Design review of the part built by this model. Coordinates are the model's own, in mm. Face numbers are marked on the shaded views. Give positions to 0.01 mm unless a question says otherwise; leave off trailing zeros. Write each loop counter-clockwise with the first axis right and the second up, starting at its lowest first coordinate (ties: lowest second). Pieces come first, ordered by that corner, then holes. Notation, with made-up numbers: (-10, -36.75) -> (13, -36.75) arc R25 ccw to (13, -22.75) -> close; hole circle Ø1 at (68.25, 70). An arc over 180 degrees is marked (long way). Return JSON: item names as keys, results as strings. Group by question number.
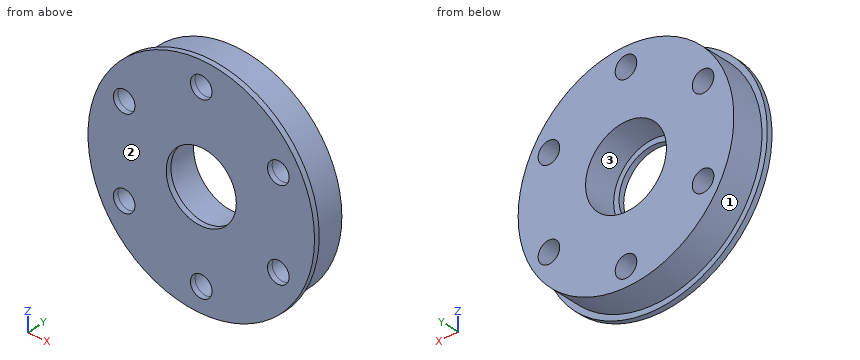
from build123d import *

# Parameters (mm, degrees)
SKETCH1_R           = 20
SKETCH1_R_2         = 7.5
BOSS_EXTRUDE1_DEPTH = 6
SKETCH2_R           = 2
CUT_EXTRUDE1_DEPTH  = 7
CIRPATTERN2_COUNT   = 6
SKETCH3_R           = 21
SKETCH3_R_2         = 6.5
SKETCH3_R_3         = 2
BOSS_EXTRUDE2_DEPTH = 1


with BuildPart() as part:
    # Sketch1 → Boss-Extrude1 (new body)
    with BuildSketch(Plane(origin=(0, 0, 0), x_dir=(1, 0, 0), z_dir=(0, 1, 0))):
        Circle(SKETCH1_R)
        Circle(SKETCH1_R_2, mode=Mode.SUBTRACT)
    extrude(amount=BOSS_EXTRUDE1_DEPTH)

    # Sketch2 → Cut-Extrude1 (cut, through all)
    with BuildSketch(Plane(origin=(0, 6, 0), x_dir=(1, 0, 0), z_dir=(0, 1, 0))):
        with Locations((0, 16.5)):
            Circle(SKETCH2_R)
    cut_extrude1 = extrude(amount=-CUT_EXTRUDE1_DEPTH, mode=Mode.SUBTRACT)

    # CirPattern2: Cut-Extrude1 ×6 about axis
    cirpattern2_axis = Axis((0, 0, 0), (0, 1, 0))
    for i in range(1, CIRPATTERN2_COUNT):
        add(cut_extrude1.rotate(cirpattern2_axis, i * 360 / CIRPATTERN2_COUNT), mode=Mode.SUBTRACT)

    # Sketch3 → Boss-Extrude2 (add)
    with BuildSketch(Plane(origin=(0, 0, 0), x_dir=(1, 0, 0), z_dir=(0, 1, 0))):
        Circle(SKETCH3_R)
        Circle(SKETCH3_R_2, mode=Mode.SUBTRACT)
        with Locations((-14.289419162, -8.25)):
            Circle(SKETCH3_R_3, mode=Mode.SUBTRACT)
        with Locations((0, -16.5)):
            Circle(SKETCH3_R_3, mode=Mode.SUBTRACT)
        with Locations((14.289419162, -8.25)):
            Circle(SKETCH3_R_3, mode=Mode.SUBTRACT)
        with Locations((14.289419162, 8.25)):
            Circle(SKETCH3_R_3, mode=Mode.SUBTRACT)
        with Locations((0, 16.5)):
            Circle(SKETCH3_R_3, mode=Mode.SUBTRACT)
        with Locations((-14.289419162, 8.25)):
            Circle(SKETCH3_R_3, mode=Mode.SUBTRACT)
    extrude(amount=-BOSS_EXTRUDE2_DEPTH)


solid = part.part
Q1. Mouldability with a two-part tool opening along Z and no side actions: class the marked faces 1, 2 and 3 as +Z half, -Z half, draft (parallel to the pull), parting line (faces both ways), or undercut.
Q2. Take a section at A-A, the plane z = 0. Give the boundary of the cut face in (x, y), plus the area to 3 significant figures.
Q3. Take a section at B-B, the plane x = 0. Give the boundary of the cut face in (y, z).
Q4. Take a section at D-D, the plane y = 4.75. Give the boundary of the cut face in (x, z), plus the area to 3 significant figures.
Q5. Take a section at C-C, the plane z = 8.25. Give the boundary of the cut face in (x, y), plus the area to 3 significant figures.
Q6. Insertion check: pin 1 (12 mm diameter, centred on x = 0, z = 0, fed in from -Y); pin 2 (1 mm diameter, centred on y = 1.5, z = 7, fed in from +X); pin 3 (4 mm diameter, centred on y = 2.5, z = -1, fed in from +X); pin 4 (1 mm diameter, centred on x = -10, y = 5, fed in from +Z). Each pin has a flat end and moves straight along its axis. Give the tip position at first contact, or say it passes through.
Q7. For L1, parallel to Z at x = 0, y = 4; L2, parallel to Z at x = -16, y = 3; L3, parallel to X at y = 3.25, z = -8.25, list the stretches that pass through material, from the lowest coordinate up. Write a range as from..to.
Final values:
{
 "1": {"face 1": "parting line", "face 2": "draft", "face 3": "undercut"},
 "2": {"outline": "(-21, -1) -> (-6.5, -1) -> (-6.5, 0) -> (-7.5, 0) -> (-7.5, 6) -> (-20, 6) -> (-20, 0) -> (-21, 0) -> close; (6.5, -1) -> (21, -1) -> (21, 0) -> (20, 0) -> (20, 6) -> (7.5, 6) -> (7.5, 0) -> (6.5, 0) -> close", "area": "179 mm²"},
 "3": {"outline": "(-1, -21) -> (0, -21) -> (0, -20) -> (6, -20) -> (6, -18.5) -> (-1, -18.5) -> close; (-1, -14.5) -> (6, -14.5) -> (6, -7.5) -> (0, -7.5) -> (0, -6.5) -> (-1, -6.5) -> close; (-1, 6.5) -> (0, 6.5) -> (0, 7.5) -> (6, 7.5) -> (6, 14.5) -> (-1, 14.5) -> close; (-1, 18.5) -> (6, 18.5) -> (6, 20) -> (0, 20) -> (0, 21) -> (-1, 21) -> close"},
 "4": {"outline": "circle Ø40 at (0, 0); hole circle Ø4 at (-14.29, -8.25); hole circle Ø4 at (-14.29, 8.25); hole circle Ø15 at (0, 0); hole circle Ø4 at (0, -16.5); hole circle Ø4 at (0, 16.5); hole circle Ø4 at (14.29, -8.25); hole circle Ø4 at (14.29, 8.25)", "area": "1,000 mm²"},
 "5": {"outline": "(-19.31, -1) -> (-16.29, -1) -> (-16.29, 6) -> (-18.22, 6) -> (-18.22, 0) -> (-19.31, 0) -> close; (-12.29, -1) -> (12.29, -1) -> (12.29, 6) -> (-12.29, 6) -> close; (16.29, -1) -> (19.31, -1) -> (19.31, 0) -> (18.22, 0) -> (18.22, 6) -> (16.29, 6) -> close", "area": "201 mm²"},
 "6": {"pin 1": "passes through", "pin 2": "stops at x = 18.91", "pin 3": "stops at x = 20", "pin 4": "stops at z = 17.6"},
 "7": {"L1": "z = -20..-18.5, -14.5..-7.5, 7.5..14.5, 18.5..20", "L2": "z = -12..-9.29, -7.21..7.21, 9.29..12", "L3": "x = -18.22..-16.29, -12.29..12.29, 16.29..18.22"}
}
